Autodesk Inventor part; units mm, degrees
ref_plane "YZ Plane" through (0, 0, 0) normal (1, 0, 0) x (0, 1, 0)
ref_plane "XZ Plane" through (0, 0, 0) normal (0, 1, 0) x (-1, 0, 0)
ref_plane "XY Plane" through (0, 0, 0) normal (0, 0, 1) x (1, 0, 0)
sketch "Sketch1" plane through (0, 0, 0) normal (0, 0, 1) x (1, 0, 0)
  line L0 (0, 0) -> (215.9, 0)
  line L1 (215.9, 0) -> (215.9, 25.4)
  line L2 (215.9, 25.4) -> (0, 25.4)
  line L3 (0, 25.4) -> (0, 0)
  dimension "d0" = 215.9
  dimension "d1" = 25.4
extrude "Extrusion1" add sketch "Sketch1" along normal blind 8.89
sketch "Sketch2" plane through (0, 0, 8.89) normal (0, 0, 1) x (1, 0, 0)
  line L0 (0, 0) -> (215.9, 0)
  line L1 (215.9, 0) -> (215.9, 25.4)
  line L2 (215.9, 25.4) -> (177.8, 25.4)
  line L3 (177.8, 25.4) -> (177.8, 0)
  line L4 (177.8, 0) -> (215.9, 0)
  line L5 (215.9, 0) -> (215.9, 25.4)
  line L6 (215.9, 25.4) -> (177.8, 25.4)
  line L7 (177.8, 25.4) -> (177.8, 12.7)
  line L8 (177.8, 12.7) -> (215.9, 12.7)
  line L9 (215.9, 12.7) -> (215.9, 25.4)
  line L10 (215.9, 25.4) -> (177.8, 25.4)
  line L11 (177.8, 25.4) -> (177.8, 19.05)
  line L12 (177.8, 19.05) -> (215.9, 19.05)
  line L13 (215.9, 19.05) -> (215.9, 25.4)
  line L14 (215.9, 0) -> (177.8, 0)
  line L15 (177.8, 0) -> (177.8, 6.35)
  line L16 (177.8, 6.35) -> (215.9, 6.35)
  line L17 (215.9, 6.35) -> (215.9, 0)
  dimension "d4" = 6.35
  dimension "d5" = 38.1
extrude "Extrusion2" add sketch "Sketch2" along normal blind 5.08 contours L3 L8 L1 L16 | L3 L12 L1 L8
sketch "Sketch3" plane through (0, 0, 13.97) normal (0, 0, 1) x (1, 0, 0)
  line L0 (215.9, 19.05) -> (177.8, 19.05)
  line L1 (177.8, 19.05) -> (177.8, 6.35)
  line L2 (177.8, 6.35) -> (215.9, 6.35)
  line L3 (215.9, 6.35) -> (215.9, 19.05)
  line L4 (215.9, 19.05) -> (177.8, 19.05)
  line L5 (177.8, 19.05) -> (177.8, 6.35)
  line L6 (215.9, 19.05) -> (177.8, 19.05)
  line L7 (177.8, 19.05) -> (177.8, 21.971)
  line L8 (177.8, 21.971) -> (215.9, 21.971)
  line L9 (215.9, 21.971) -> (215.9, 19.05)
  line L10 (215.9, 6.35) -> (177.8, 6.35)
  line L11 (177.8, 6.35) -> (177.8, 3.429)
  line L12 (177.8, 3.429) -> (215.9, 3.429)
  line L13 (215.9, 3.429) -> (215.9, 6.35)
  point P0 (0, 0)
  dimension "d8" = 2.921
  dimension "d9" = 2.921
extrude "Extrusion3" add sketch "Sketch3" along normal blind 5.08
sketch "Sketch4" plane through (0, 0, 0) normal (0, 0, -1) x (-1, 0, 0)
  circle A0 centre (-202.0681, 12.7) radius 4.445
  dimension "d12" = 8.89
extrude "Extrusion4" cut sketch "Sketch4" against normal blind 127
sketch "Sketch5" plane through (0, 0, 8.89) normal (0, 0, 1) x (1, 0, 0)
  circle A0 centre (15.8377, 12.7) radius 6.35
  dimension "d17" = 12.7
extrude "Extrusion5" cut sketch "Sketch5" against normal blind 25.4
properties part number "Piece One-Diagonal Piece" material "Steel"
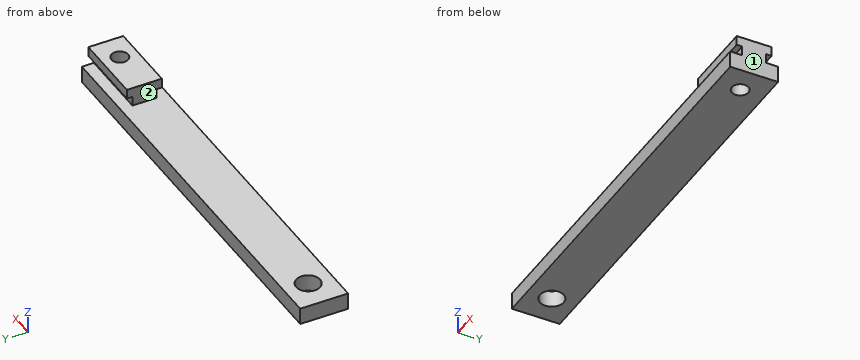
The listing builds one solid part. Answer for the finished solid, in the listing's coordinates (mm). Face numbers are marked on the shaded views. A direction names the side the tool comes from. Give positions to 0.01 mm unless a question says otherwise; leave off trailing zeros. Loops run counter-clockwise (first coordinate to the right, second up) from the corner with the lowest first, then second, coordinate; pieces in that order, holes last. Notation, with made-up numbers: M 20.25,-0.5 L 31.25,-0.5 A17 cw 31.25,6.5 Z; hole C 31.5,-40 d11. An arc over 180 degrees is marked long. One line per item, written item: value.
1. For the marked faces 1 and 2, determine the directions among +Z, -Z, +X, -X, +Y, -Y from which every point of the face is accessible in a straight line to the end or side of a thin tool.
Found:
face 1: +Z, -Z, +X, +Y, -Y
face 2: +Z, -X, +Y, -Y
2. Section D-D on x = 96 is taken. Determine the outline of the cut face in (y, z), plus the area to 3 significant figures.
Found:
outline: M 0,0 L 25.4,0 L 25.4,8.89 L 0,8.89 Z
area: 226 mm^2
3. Find the intervals of material crossed by probe 1 along X at (y, z) = (15.5, 8); probe 2 along X at (y, z) = (9.75, 4.5); probe 3 along Z at (x, y) = (100.5, 24), in increasing order.
Found:
probe 1: 0 to 10.14, 21.54 to 198.62, 205.52 to 215.9
probe 2: 0 to 10.21, 21.46 to 198.74, 205.39 to 215.9
probe 3: 0 to 8.89
4. Section A-A on y = 12.7 is taken. Determine the outline of the cut face in (x, z), plus the area to 3 significant figures.
Found:
outline: M 0,0 L 9.49,0 L 9.49,8.89 L 0,8.89 Z; M 22.19,0 L 197.62,0 L 197.62,19.05 L 177.8,19.05 L 177.8,8.89 L 22.19,8.89 Z; M 206.51,0 L 215.9,0 L 215.9,19.05 L 206.51,19.05 Z
area: 2,020 mm^2
5. Section C-C on z = 4.5 is taken. Determine the outline of the cut face in (x, y) (3 decimals).
Found:
outline: M 0,0 L 215.9,0 L 215.9,25.4 L 0,25.4 Z; hole C 15.838,12.7 d12.7; hole C 202.068,12.7 d8.89
6. Section B-B on z = 17 is taken. Determine the outline of the cut face in (x, y) (3 decimals).
Found:
outline: M 177.8,3.429 L 215.9,3.429 L 215.9,21.971 L 177.8,21.971 Z; hole C 202.068,12.7 d8.89
7. Each of these flat-tipped pins is pushed along its axis until it touches: P1, Ø5.5, axis at x = 202.07, y = 12.7, coming from the +Z side; P2, Ø1.5, axis at x = 190, z = 16.5, coming from the +Y side; P3, Ø2, axis at x = 82.5, z = 8.5, coming from the -Y side; P4, Ø10, axis at y = 6, z = 14.5, coming from the -X side. Where does it stop, or does it pass through?
Found:
P1: through
P2: y = 21.97
P3: y = 0
P4: x = 177.8
